Part model, mm, in its own coordinate system. A direction names the side the tool comes from. Coordinates: 2 decimals unless noted, no trailing zeros. Order: outer loops, then holes, each group sorted by start corner. A loop starts at its lowest first (then second) coordinate and runs counter-clockwise, first axis right, second up. Notation, with made-up numbers: (-27, 2) - (24, 2) arc R21 cw to (24, 7) - close; hole circle Ø6 at (-33, 71.25). An arc over 180 degrees is marked (long way). Use a Markdown table: item, result. Add a question column.
1) Wall check: L1, parallel to Z at x = 0, y = -7.5; L2, parallel to Y at x = -4, z = -3.75; L3, parallel to Z at x = 0, y = 6.25. Give the ranges that are in metal, low to high. Write a range as [from, to].
2) Saw through at D-D on y = -3.5. List the corners of the cut face in (x, z), then the cut area to 3 significant figures.
3) Saw through at C-C on x = -8. List the corners of the cut face in (y, z), then the cut area to 3 significant figures.
4) Saw through at A-A on z = 0. List the corners of the cut face in (x, y).
5) Two-plate mould, pull along Z, no slides. Class faces 1 (the face through (-12, 9, -2)), 2 (the face through (-1.487, -7.204, 0.195)), 3 (the face through (-11.99, -0.13, 0.53)): +Z half, -Z half, draft (parallel to the pull), parting line (faces both ways), or undercut.
6) Saw through at B-B on x = 10.75. List the corners of the cut face in (y, z).
7) Tool access for faces 4 (the face through (-9, 10.5, -3)), 5 (the face through (6.08, -6.95, 1.43)), 6 (the face through (-12, -9, -2)), 7 (the face through (0, -4, 2)): list every direction of +Z, -Z, +X, -X, +Y, -Y with a clear straight run to the whole face (end or side of a thin tool).
8) Drop flat-ended pins along their axis: P1, Ø12, axis at x = 3, z = 7, coming from the +Y side; P2, Ø4, axis at y = 6, z = 6, coming from the +X side; P3, Ø6, axis at y = -6.5, z = -8, coming from the +X side; P4, Ø1.5, axis at x = -4.5, y = 5.5, coming from the +Z side. Give the stop position or say it passes through.
Autodesk Inventor part; units mm, degrees
ref_plane "YZ Plane" through (0, 0, 0) normal (1, 0, 0) x (0, 1, 0)
ref_plane "XZ Plane" through (0, 0, 0) normal (0, 1, 0) x (-1, 0, 0)
ref_plane "XY Plane" through (0, 0, 0) normal (0, 0, 1) x (1, 0, 0)
sketch "Náčrt1" plane through (0, 0, 0) normal (0, 1, 0) x (-1, 0, 0)
  circle A0 centre (0, 0) radius 16.5
  circle A1 centre (0, 0) radius 13.5
  dimension "d0" = 33
  dimension "d1" = 27
extrude "Vysunutí1" add sketch "Náčrt1" along normal mid plane 21 contours A1
sketch "Náčrt4" plane through (0, 0, 0) normal (1, 0, 0) x (0, 1, 0)
  line L0 (-10.5, 13.5) -> (-10.5, -13.5)
  point P0 (0, 0)
  point P1 (-6.5, 0)
  dimension "d16" = 4
hole "Díra2" at (0, -6.5, 0) direction (1, 0, 0) diameter 3 end through all
thread "Závit1"
extrude "Vysunutí2" add sketch "Náčrt1" along normal mid plane 18
sketch "Náčrt2" plane through (0, 10.5, 0) normal (0, 1, 0) x (1, 0, 0)
  circle A0 centre (0, 0) radius 9
  dimension "d6" = 18
extrude "Vysunutí3" cut sketch "Náčrt2" against normal blind 14.5
sketch "Náčrt3" plane through (0, -10.5, 0) normal (0, -1, 0) x (1, 0, 0)
  circle A0 centre (0, 0) radius 13.5
hole "Díra1" at (0, -10.5, 0) direction (0, 1, 0) diameter 3 end through all
sketch "Náčrt5" plane through (0, -9, 0) normal (0, -1, 0) x (1, 0, 0)
  circle A0 centre (0, 0) radius 16.5
  circle A1 centre (0, 0) radius 1.5
  circle A2 centre (0, 0) radius 12
  dimension "d26" = 24
extrude "Vysunutí4" cut sketch "Náčrt5" against normal up to surface (18 mm away) contours A0
properties part number "JSUMO_Wheel_33x20mm_NoSilicon"
Results are:
| question | item | result |
|---|---|---|
| 1 | L1 | [-12, -1.5], [1.5, 12] |
| 1 | L2 | [-10.5, -4] |
| 1 | L3 | [-12, -9], [9, 12] |
| 2 | outline | circle Ø24 at (0, 0); hole circle Ø18 at (0, 0) |
| 2 | area | 198 mm2 |
| 3 | outline | (-10.5, -10.87) - (-9, -10.87) - (-9, -8.94) - (9, -8.94) - (9, -10.87) - (10.5, -10.87) - (10.5, -4.12) - (-4, -4.12) - (-4, 4.12) - (10.5, 4.12) - (10.5, 10.87) - (9, 10.87) - (9, 8.94) - (-9, 8.94) - (-9, 10.87) - (-10.5, 10.87) - close |
| 3 | area | 268 mm2 |
| 4 | outline | (-13.5, -10.5) - (-1.5, -10.5) - (-1.5, -4) - (-9, -4) - (-9, 10.5) - (-13.5, 10.5) - (-13.5, 9) - (-12, 9) - (-12, -9) - (-13.5, -9) - close; (1.5, -10.5) - (13.5, -10.5) - (13.5, -9) - (12, -9) - (12, -8) - (1.5, -8) - close; (1.5, -5) - (12, -5) - (12, 9) - (13.5, 9) - (13.5, 10.5) - (9, 10.5) - (9, -4) - (1.5, -4) - close |
| 5 | face 1 | draft |
| 5 | face 2 | undercut |
| 5 | face 3 | parting line |
| 6 | outline | (-10.5, -8.17) - (-9, -8.17) - (-9, -5.33) - (9, -5.33) - (9, -8.17) - (10.5, -8.17) - (10.5, 8.17) - (9, 8.17) - (9, 5.33) - (-9, 5.33) - (-9, 8.17) - (-10.5, 8.17) - close; hole circle Ø3 at (-6.5, 0) |
| 7 | face 4 | +Z, -Z, +X, -X, +Y |
| 7 | face 5 | +X |
| 7 | face 6 | none |
| 7 | face 7 | +Y |
| 8 | P1 | y = 10.5 |
| 8 | P2 | x = 11.31 |
| 8 | P3 | x = 11.92 |
| 8 | P4 | z = 11.4 |
